Autodesk Inventor part; units mm, degrees
ref_plane "YZ Plane" through (0, 0, 0) normal (1, 0, 0) x (0, 1, 0)
ref_plane "XZ Plane" through (0, 0, 0) normal (0, 1, 0) x (-1, 0, 0)
ref_plane "XY Plane" through (0, 0, 0) normal (0, 0, 1) x (1, 0, 0)
sketch "Sketch1" plane through (0, 0, 0) normal (0, 1, 0) x (-1, 0, 0)
  line L0 (8.9115, 17.7017) -> (-16.4885, 17.7017)
  line L1 (-16.4885, 17.7017) -> (-16.4885, -33.0983)
  line L2 (-16.4885, -33.0983) -> (8.9115, -33.0983)
  line L3 (8.9115, -33.0983) -> (8.9115, 17.7017)
  line L4 (8.9115, 17.7017) -> (2.5615, 17.7017)
  line L5 (2.5615, 17.7017) -> (2.5615, 5.0017)
  line L6 (2.5615, 5.0017) -> (8.9115, 5.0017)
  line L7 (8.9115, 5.0017) -> (8.9115, 17.7017)
  line L8 (-16.4885, 17.7017) -> (-10.1385, 17.7017)
  line L9 (-10.1385, 17.7017) -> (-10.1385, 5.0017)
  line L10 (-10.1385, 5.0017) -> (-16.4885, 5.0017)
  line L11 (-16.4885, 5.0017) -> (-16.4885, 17.7017)
  line L12 (8.9115, -33.0983) -> (2.5615, -33.0983)
  line L13 (2.5615, -33.0983) -> (2.5615, -20.3983)
  line L14 (2.5615, -20.3983) -> (8.9115, -20.3983)
  line L15 (8.9115, -20.3983) -> (8.9115, -33.0983)
  line L16 (-16.4885, -33.0983) -> (-10.1385, -33.0983)
  line L17 (-10.1385, -33.0983) -> (-10.1385, -20.3983)
  line L18 (-10.1385, -20.3983) -> (-16.4885, -20.3983)
  line L19 (-16.4885, -20.3983) -> (-16.4885, -33.0983)
  circle A0 centre (-3.7885, -7.6983) radius 4.1275
  point P0 (0, 0)
  dimension "d0" = 25.4
  dimension "d1" = 50.8
  dimension "d2" = 6.35
  dimension "d3" = 12.7
  dimension "d4" = 6.35
  dimension "d5" = 12.7
  dimension "d6" = 6.35
  dimension "d7" = 12.7
  dimension "d8" = 6.35
  dimension "d9" = 12.7
  dimension "d10" = 8.255
extrude "Extrusion1" add sketch "Sketch1" against normal blind 12.7 contours L5 L6 L3 L14 L13 L2 L17 L18 L1 L10 L9 L0
sketch "Sketch2" plane through (10.1385, -12.7, 17.7017) normal (1, 0, 0) x (0, 0, -1)
  circle A0 centre (6.35, 6.35) radius 2.5083
  line L0 (0, 0) -> (0, 12.7)
  line L1 (12.7, 0) -> (0, 0)
  circle A1 centre (44.45, 6.35) radius 2.5083
  line L2 (38.1, 12.7) -> (50.8, 12.7)
  line L3 (50.8, 12.7) -> (50.8, 0)
  point P0 (17.7017, 12.7)
  dimension "d13" = 5.0165
  dimension "d14" = 6.35
  dimension "d15" = 6.35
  dimension "d16" = 5.0165
  dimension "d17" = 6.35
  dimension "d18" = 6.35
extrude "Extrusion2" cut sketch "Sketch2" against normal blind 12.7
fillet "Fillet1" radius 6.35 4 edges at (3.7885, 0, 17.7017) (3.7885, -12.7, 17.7017) (3.7885, 0, -33.0983) (3.7885, -12.7, -33.0983)
sketch "Sketch3" plane through (0, 0, 0) normal (0, 1, 0) x (1, 0, 0)
  circle A0 centre (-6.8795, -2.9697) radius 1.397
  line L0 (-8.9115, -5.0017) -> (-2.5615, -5.0017)
  line L1 (-8.9115, 20.3983) -> (-8.9115, -5.0017)
  circle A1 centre (14.4565, -2.9697) radius 1.397
  line L2 (16.4885, -5.0017) -> (16.4885, 20.3983)
  circle A2 centre (14.4565, 18.3663) radius 1.397
  line L3 (16.4885, 20.3983) -> (10.1385, 20.3983)
  circle A3 centre (-6.8795, 18.3663) radius 1.397
  point P0 (0, 0)
  dimension "d22" = 2.794
  dimension "d23" = 2.032
  dimension "d24" = 2.032
  dimension "d25" = 2.794
  dimension "d26" = 2.032
  dimension "d27" = 2.794
  dimension "d28" = 2.032
  dimension "d29" = 2.794
extrude "Extrusion3" cut sketch "Sketch3" against normal blind 7.62
sketch "Sketch4" plane through (0, 0, 0) normal (0, 1, 0) x (1, 0, 0)
  line L0 (2.6455, 1.0308) -> (4.9315, 1.0308)
  line L1 (4.9315, 1.0308) -> (4.9315, 3.7322)
  line L2 (2.6455, 3.7322) -> (2.6455, 1.0308)
  circle A0 centre (3.7885, 7.6983) radius 4.1275
  line L3 (4.9315, 14.3658) -> (2.6455, 14.3658)
  line L4 (2.6455, 14.3658) -> (2.6455, 11.6644)
  line L5 (4.9315, 11.6644) -> (4.9315, 14.3658)
  point P0 (0, 0)
  dimension "d32" = 2.286
  dimension "d34" = 8.255
  dimension "d36" = 1.143
  dimension "d37" = 2.286
extrude "Extrusion4" cut sketch "Sketch4" against normal blind 2.286 contours L2 A0 L1 L0 | L4 L3 L5 A0
properties part number "bottom_anchor_v3"
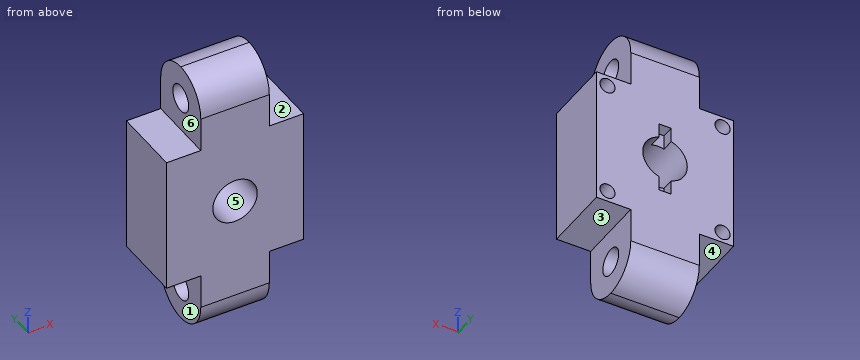
Geometry check sheet. Reference: the model listing, model coordinates, mm. Face numbers are marked on the shaded views. A direction names the side the tool comes from. Round coordinates to 2 decimals unless told otherwise and drop trailing zeros. Order: outer loops, then holes, each group sorted by start corner. A loop starts at its lowest first (then second) coordinate and runs counter-clockwise, first axis right, second up. Notation, with made-up numbers: M 81.25,80.5 L 96.25,80.5 A12 cw 96.25,95.5 Z; hole C -8.5,67.5 d2. An arc over 180 degrees is marked long. Answer in a Markdown table with one row per item. Add a question column.
Item 1: Material ranges on L1, parallel to X at y = -0.5, z = 3; L2, parallel to Y at x = 7.25, z = 11.5; L3, parallel to X at y = -7.25, z = -19, recorded low to high. Write a range as [from, to].
Item 2: Sectioned sample at B-B, the plane z = 12.5. Enter the section's corners in (x, y), plus the area to 3 significant figures.
Item 3: Draft check along X on the marked faces 4, 5 and 6. Enter one of: released by +X, released by -X, zero draft, split by the parting line, or undercut.
Item 4: Sectioned sample at C-C, the plane x = -6.5. Enter the section's corners in (y, z), plus the area to 3 significant figures.
Item 5: Set-up check for the marked faces 1, 2 and 3: record each of +Z, -Z, +X, -X, +Y, -Y from which the full face is reachable in a straight line by a thin tool's end or side.
Item 6: Sectioned sample at A-A, the plane y = -5.5. Enter the section's corners in (x, z) (1 decimal), plus the area to 3 significant figures.
Item 7: Depth check by flat-ended pin: pin 1 Ø1.1 at (x, y) = (3.5, -1) entering from +Z; pin 2 Ø1.8 at (x, z) = (4, -2) entering from +Y; pin 3 Ø1.8 at (x, y) = (3, -1.5) entering from -Z; pin 4 Ø4.5 at (y, z) = (-6.35, 11.35) entering from +X. Enter the tip coordinate at first touch or a pass-through.
Item 8: Sectioned sample at D-D, the plane x = 13.75. Enter the section's corners in (y, z).
Filled in:
| question | item | result |
|---|---|---|
| 1 | L1 | x = [-8.91, -8.28], [-5.48, 13.06], [15.85, 16.49] |
| 1 | L2 | y = [-12.7, -8.85], [-3.85, 0] |
| 1 | L3 | x = [-8.91, -8.12], [-5.63, 13.21], [15.7, 16.49] |
| 2 | outline | M -2.56,-12.6 L 10.14,-12.6 L 10.14,-8.58 L -2.56,-8.58 Z; M -2.56,-4.12 L 10.14,-4.12 L 10.14,-0.1 L -2.56,-0.1 Z |
| 2 | area | 102 mm² |
| 3 | face 4 | zero draft |
| 3 | face 5 | undercut |
| 3 | face 6 | released by -X |
| 4 | outline | M -12.7,-20.4 L 0,-20.4 L 0,-19.71 L -7.62,-19.71 L -7.62,-17.02 L 0,-17.02 L 0,1.63 L -7.62,1.63 L -7.62,4.31 L 0,4.31 L 0,5 L -12.7,5 Z |
| 4 | area | 282 mm² |
| 5 | face 1 | -Z, -X, +Y, -Y |
| 5 | face 2 | +Z, +X, +Y, -Y |
| 5 | face 3 | -Z, +X, +Y, -Y |
| 6 | outline | M -8.9,-20.4 L -2.6,-20.4 L -2.6,-24.4 L 10.1,-24.4 L 10.1,-20.4 L 16.5,-20.4 L 16.5,5 L 10.1,5 L 10.1,9 L -2.6,9 L -2.6,5 L -8.9,5 Z; M -2.6,-33 L 10.1,-33 L 10.1,-29.1 L -2.6,-29.1 Z; M -2.6,13.7 L 10.1,13.7 L 10.1,17.6 L -2.6,17.6 Z; hole C -6.9,-18.4 d2.8; hole C -6.9,3 d2.8; hole C 3.8,-7.7 d8.3; hole C 14.5,-18.4 d2.8; hole C 14.5,3 d2.8 |
| 6 | area | 768 mm² |
| 7 | pin 1 | stops at z = 15.51 |
| 7 | pin 2 | stops at y = -2.29 |
| 7 | pin 3 | stops at z = -31.72 |
| 7 | pin 4 | passes through |
| 8 | outline | M -12.7,-20.4 L 0,-20.4 L 0,-19.57 L -7.62,-19.57 L -7.62,-17.16 L 0,-17.16 L 0,1.76 L -7.62,1.76 L -7.62,4.17 L 0,4.17 L 0,5 L -12.7,5 Z |
